Verification items for the finished model (mm, model axes). A direction names the side the tool comes from. Round coordinates to 2 decimals unless told otherwise and drop trailing zeros. Order: outer loops, then holes, each group sorted by start corner. A loop starts at its lowest first (then second) coordinate and runs counter-clockwise, first axis right, second up. Notation, with made-up numbers: M 83,80 L 108,80 A13 cw 108,91 Z; hole C 53.5,19 d4. An arc over 180 degrees is marked long. Use CSV: the item, a comma, the result in double quotes. Start each with the question number.
Q1. Set-up check for faces 4 (the face through (-12.52, -3.338, 0.147)), 5 (the face through (20.15, 28.84, 0.37)), 6 (the face through (17.531, -1.4, 31.9)), 7 (the face through (22.368, -4.686, 35.694)): record each of +Z, -Z, +X, -X, +Y, -Y from which the full face is reachable in a straight line by a thin tool's end or side.
Q2. Sectioned sample at D-D (x = 11.5). Enter the section's corners in (y, z), and give its area (3 significant figures).
Q3. Mould release check, pull along Y, two halves, no side actions. Record for faces 1 (the face through (19.368, -5.077, 38.668)), 2 (the face through (-18.509, 2.1, 0)), 3 (the face through (20.15, 0.51, -32.12)): +Y half, -Y half, draft (parallel to the pull), parting line (faces both ways), or undercut.
Q4. Sectioned sample at A-A (z = 0). State how many separate pieces and enclosed holes the cut face has, and give its area (3 significant figures).
Q5. Scan lines: line 1 (Y direction, x = 14.9, z = 0); line 2 (X direction, y = -19, z = -24); line 3 (Y direction, x = 19.4, z = 30.5). Record each from-to range of solid material in increasing order.
Q6. Gauge pin test, flat ends, axial feed: pin 1 Ø1 at (y, z) = (-5.5, 28.5) entering from -X; pin 2 Ø3.5 at (y, z) = (0, -1) entering from +X; pin 3 Ø4 at (y, z) = (0, 30.5) entering from -X; pin 4 Ø2.5 at (y, z) = (-30.5, 0) entering from +X. Record the tip position at first contact, or that the pin passes through.
Q7. Sectioned sample at C-C (x = -7). Enter the section's corners in (y, z), and give its area (3 significant figures).
```python
from build123d import *

# Parameters (mm, degrees)
SKETCH1_W                                           = 0.566
SKETCH1_H                                           = 1
CBORE_FOR_M3_HEX_SOCKET_HEAD_CAP_SCREW2_D           = 3.4
CBORE_FOR_M3_HEX_SOCKET_HEAD_CAP_SCREW2_DEPTH       = 8.566
CBORE_FOR_M3_HEX_SOCKET_HEAD_CAP_SCREW2_CBORE_D     = 6.5
CBORE_FOR_M3_HEX_SOCKET_HEAD_CAP_SCREW2_CBORE_DEPTH = 3.4
CBORE_FOR_M3_HEX_SOCKET_HEAD_CAP_SCREW2_TIP         = 1.021463052
CHAMFER1_SIZE                                       = 2


with BuildPart() as part:
    # Sketch1 → Revolve17 (revolve)
    with BuildSketch(Plane.XY):
        Polygon((-14.175209939, 3.15), (-14.175209939, 3.65), (-18.508543272, 3.15), (-18.508543272, 1.9), (0, 1.9), (21.56511535, 21.5), (22.13111535, 21.5), (22.13111535, 22.5), (22.13111535, 24.5), (22.69711535, 24.5), (22.69711535, 34), (22.03011535, 34), (22.03011535, 36), (22.69711535, 36), (22.69711535, 39), (14.13111535, 39), (14.13111535, 21.5), (-5.508543272, 3.65), (-9.841876606, 3.15), (-9.841876606, 3.65), align=None)
        with Locations((22.41411535, 22)):
            Rectangle(SKETCH1_W, SKETCH1_H)
    revolve(axis=Axis((-801.920554309, 0, 0), (1, 0, 0)))

    # CBORE for M3 Hex Socket Head Cap Screw2
    with Locations(Plane.ZY.offset(-14.13111535)):
        with Locations((0, -30.5), (0, 30.5), (30.5, 0), (-30.5, 0)):
            CounterBoreHole(CBORE_FOR_M3_HEX_SOCKET_HEAD_CAP_SCREW2_D / 2, CBORE_FOR_M3_HEX_SOCKET_HEAD_CAP_SCREW2_CBORE_D / 2, CBORE_FOR_M3_HEX_SOCKET_HEAD_CAP_SCREW2_CBORE_DEPTH, depth=CBORE_FOR_M3_HEX_SOCKET_HEAD_CAP_SCREW2_DEPTH)
            with Locations((0, 0, -(CBORE_FOR_M3_HEX_SOCKET_HEAD_CAP_SCREW2_DEPTH + CBORE_FOR_M3_HEX_SOCKET_HEAD_CAP_SCREW2_TIP / 2))):  # 118° drill point
                Cone(0, CBORE_FOR_M3_HEX_SOCKET_HEAD_CAP_SCREW2_D / 2, CBORE_FOR_M3_HEX_SOCKET_HEAD_CAP_SCREW2_TIP, mode=Mode.SUBTRACT)

    # Chamfer1
    chamfer1_edges = [part.edges().sort_by_distance(p)[0] for p in [
        (14.13111535, -39, 0),
    ]]
    chamfer(chamfer1_edges, length=CHAMFER1_SIZE)


solid = part.part
```
Verdict:
1,face 4,"none"
1,face 5,"+X, -X"
1,face 6,"-X"
1,face 7,"+X"
2,outline,"C 0,0 d38.22; hole C 0,0 d24.7"
2,area,"668 mm²"
3,face 1,"parting line"
3,face 2,"draft"
3,face 3,"undercut"
4,separate pieces,"4"
4,enclosed holes,"0"
4,area,"539 mm²"
5,line 1,"y = -37.77 to -33.75, -27.25 to -15.44, 15.44 to 27.25, 33.75 to 37.77"
5,line 2,"x = 14.13 to 22.7"
5,line 3,"y = -24.31 to -1.7, 1.7 to 24.31"
6,pin 1,"stops at x = 14.13"
6,pin 2,"stops at x = 0.94"
6,pin 3,"stops at x = 17.53"
6,pin 4,"passes through"
7,outline,"C 0,0 d6.96; hole C 0,0 d3.8"
7,area,"26.7 mm²"
